Work out the finished part from the listing and answer in its coordinate system (mm). Face numbers are marked on the shaded views. Give positions to 0.01 mm unless a question says otherwise; leave off trailing zeros. Loops run counter-clockwise (first coordinate to the right, second up) from the corner with the lowest first, then second, coordinate; pieces in that order, holes last. Notation, with made-up numbers: (-1, -4.75) - (51, -4.75) arc R19 cw to (51, 28.25) - close; hole circle Ø5 at (23, 51.5). An arc over 180 degrees is marked (long way). One line per item, written item: value.
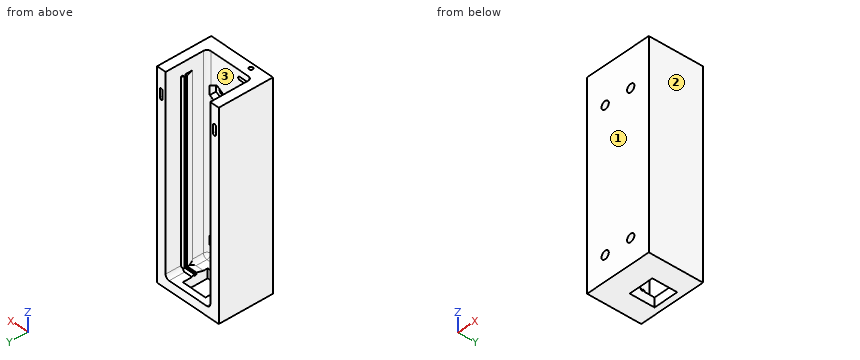
from build123d import *

# Parameters (mm, degrees)
BOSS_EXTRUDE1_DEPTH            = 82.55
BOSS_EXTRUDE2_START            = -5.08
BOSS_EXTRUDE2_DEPTH            = 77.47
BOSS_EXTRUDE4_REACH            = 89.467
SKETCH8_W                      = 27.6225
SKETCH8_H                      = 3.81
BOSS_EXTRUDE5_REACH            = 88.945
CUT_EXTRUDE1_REACH             = 86.753
SKETCH10_W                     = 10.16
SKETCH10_H                     = 10.16
SKETCH11_W                     = 27.6225
SKETCH11_H                     = 3.2766
CUT_EXTRUDE2_DEPTH             = 85.753025619
FILLET3_R                      = 1.5875
CUT_EXTRUDE3_DEPTH             = 2.286
CUT_EXTRUDE4_DEPTH             = 3.175
F_4_CLEARANCE_HOLE1_D          = 3.2639
CUT_EXTRUDE5_DEPTH             = 2.54
CUT_EXTRUDE5_DIRECTION_2_REACH = 87.415
SKETCH18_R                     = 0.762
CUT_EXTRUDE6_DEPTH             = 10.16


with BuildPart() as part:
    # Sketch1 → Boss-Extrude1 (new body)
    with BuildSketch(Plane.XY):
        Polygon((10.00125, 12.065), (10.00125, -8.255), (-10.00125, -8.255), (-10.00125, 12.065), (-13.81125, 12.065), (-13.81125, -13.335), (13.81125, -13.335), (13.81125, 12.065), align=None)
    extrude(amount=BOSS_EXTRUDE1_DEPTH)

    # Sketch3 → Boss-Extrude2 (add)
    with BuildSketch(Plane.XY.offset(82.55).offset(BOSS_EXTRUDE2_START)):
        Polygon((10.00125, 1.7018), (9.23925, 1.7018), (10.00125, 2.4638), align=None)
        Polygon((10.00125, 0.635), (9.23925, 0.635), (10.00125, -2.208822715), align=None)
        Polygon((-10.00125, 2.4638), (-10.00125, 1.7018), (-9.23925, 1.7018), align=None)
        Polygon((-10.00125, -2.208822715), (-10.00125, 0.635), (-9.23925, 0.635), align=None)
    extrude(amount=-BOSS_EXTRUDE2_DEPTH)

    # Boss-Extrude4: up to this face of the body (flat: up to its plane)
    boss_extrude4_end = Plane(part.part.faces().sort_by_distance((0, -8.255, 41.275))[0])
    # Sketch8 → Boss-Extrude4 (add, up to the picked face)
    with BuildSketch(Plane(origin=(0, 12.065, 0), x_dir=(1, 0, 0), z_dir=(0, 1, 0)), mode=Mode.PRIVATE) as boss_extrude4_sk1:
        with Locations((0, -1.905)):
            Rectangle(SKETCH8_W, SKETCH8_H)
    boss_extrude4_tool1 = split(extrude(boss_extrude4_sk1.sketch, amount=-BOSS_EXTRUDE4_REACH, mode=Mode.PRIVATE), bisect_by=boss_extrude4_end, keep=Keep.BOTH, mode=Mode.PRIVATE)
    add(boss_extrude4_tool1.solids().sort_by(Axis((0, 12.065, 1.905), (0, -1, 0)))[0])

    # Boss-Extrude5: up to this face of the body (flat: up to its plane)
    boss_extrude5_end = Plane(part.part.faces().sort_by_distance((10.00125, 7.2644, 4.623196778))[0])
    # Sketch9 → Boss-Extrude5 (add, up to the picked face)
    with BuildSketch(Plane(origin=(-10.00125, 0, 0), x_dir=(0, 0, -1), z_dir=(1, 0, 0)), mode=Mode.PRIVATE) as boss_extrude5_sk1:
        Polygon((-3.81, 2.4638), (-3.81, 1.7018), (-4.572, 1.7018), align=None)
    boss_extrude5_tool1 = split(extrude(boss_extrude5_sk1.sketch, amount=BOSS_EXTRUDE5_REACH, mode=Mode.PRIVATE), bisect_by=boss_extrude5_end, keep=Keep.BOTH, mode=Mode.PRIVATE)
    # Sketch9 → Boss-Extrude5 (add, up to the picked face)
    with BuildSketch(Plane(origin=(-10.00125, 0, 0), x_dir=(0, 0, -1), z_dir=(1, 0, 0)), mode=Mode.PRIVATE) as boss_extrude5_sk2:
        Polygon((-3.81, 0.635), (-3.81, -2.208822715), (-4.572, 0.635), align=None)
    boss_extrude5_tool2 = split(extrude(boss_extrude5_sk2.sketch, amount=BOSS_EXTRUDE5_REACH, mode=Mode.PRIVATE), bisect_by=boss_extrude5_end, keep=Keep.BOTH, mode=Mode.PRIVATE)
    add(boss_extrude5_tool1.solids().sort_by(Axis((-10.00125, 1.9558, 4.064), (1, 0, 0)))[0])
    add(boss_extrude5_tool2.solids().sort_by(Axis((-10.00125, -0.312941, 4.064), (1, 0, 0)))[0])

    # Sketch10 → Cut-Extrude1 (cut, up to next)
    with BuildSketch(Plane(origin=(0, 0, 0), x_dir=(-1, 0, 0), z_dir=(0, 0, -1)), mode=Mode.PRIVATE) as cut_extrude1_sk1:
        with Locations((0, 1.1684)):
            Rectangle(SKETCH10_W, SKETCH10_H)
    cut_extrude1_tool1 = extrude(cut_extrude1_sk1.sketch, amount=-CUT_EXTRUDE1_REACH, mode=Mode.PRIVATE) & part.part
    add(cut_extrude1_tool1.solids().sort_by_distance((0, 1.1684, 0))[0], mode=Mode.SUBTRACT)

    # Sketch11 → Cut-Extrude2 (cut, through all)
    with BuildSketch(Plane.XY.offset(82.55)):
        with Locations((0, 10.4267)):
            Rectangle(SKETCH11_W, SKETCH11_H)
    extrude(amount=-CUT_EXTRUDE2_DEPTH, mode=Mode.SUBTRACT)

    # Fillet3
    fillet3_edges = [part.edges().sort_by_distance(p)[0] for p in [
        (-10.00125, -8.255, 43.18),
        (10.00125, -8.255, 43.18),
        (10.00125, 5.6261, 3.81),
        (0, -8.255, 3.81),
        (10.00125, -5.231911358, 3.81),
        (-10.00125, 5.6261, 3.81),
        (-10.00125, -5.231911358, 3.81),
    ]]
    fillet(fillet3_edges, radius=FILLET3_R)

    # Sketch13 → Cut-Extrude3 (cut)
    with BuildSketch(Plane(origin=(0, -8.255, 0), x_dir=(1, 0, 0), z_dir=(0, 1, 0))):
        with BuildLine():
            Line((-7.651886934, -78.8162), (-4.476886934, -78.8162))
            ThreePointArc((-4.476886934, -78.8162), (-3.841886934, -79.4512), (-4.476886934, -80.0862))
            Line((-4.476886934, -80.0862), (-7.651886934, -80.0862))
            ThreePointArc((-7.651886934, -80.0862), (-8.286886934, -79.4512), (-7.651886934, -78.8162))
        make_face()
    extrude(amount=-CUT_EXTRUDE3_DEPTH, mode=Mode.SUBTRACT)

    # Sketch14 → Cut-Extrude4 (cut)
    with BuildSketch(Plane(origin=(0, 8.7884, 0), x_dir=(1, 0, 0), z_dir=(0, 1, 0))):
        with BuildLine():
            Line((-11.27125, -71.386954), (-11.27125, -74.561954))
            ThreePointArc((-11.27125, -74.561954), (-11.90625, -75.196954), (-12.54125, -74.561954))
            Line((-12.54125, -74.561954), (-12.54125, -71.386954))
            ThreePointArc((-12.54125, -71.386954), (-11.90625, -70.751954), (-11.27125, -71.386954))
        make_face()
        with BuildLine():
            Line((11.27125, -71.386954), (11.27125, -74.561954))
            ThreePointArc((11.27125, -74.561954), (11.90625, -75.196954), (12.54125, -74.561954))
            Line((12.54125, -74.561954), (12.54125, -71.386954))
            ThreePointArc((12.54125, -71.386954), (11.90625, -70.751954), (11.27125, -71.386954))
        make_face()
    extrude(amount=-CUT_EXTRUDE4_DEPTH, mode=Mode.SUBTRACT)

    # #4 Clearance Hole1 (through all)
    with Locations(Plane(origin=(0, -8.255, 0), x_dir=(1, 0, 0), z_dir=(0, 1, 0))):
        with Locations((-5.715, -10.16), (5.715, -67.31), (-5.715, -67.31), (5.715, -10.16)):
            Hole(F_4_CLEARANCE_HOLE1_D / 2)

    # Sketch17 → Cut-Extrude5 (cut)
    with BuildSketch(Plane(origin=(0, -8.255, 0), x_dir=(1, 0, 0), z_dir=(0, 1, 0))):
        Polygon((-5.715, -13.782180119), (-2.5781, -11.971090059), (-2.5781, -8.348909941), (-5.715, -6.537819881), (-8.8519, -8.348909941), (-8.8519, -11.971090059), align=None)
        Polygon((5.715, -13.782180119), (8.8519, -11.971090059), (8.8519, -8.348909941), (5.715, -6.537819881), (2.5781, -8.348909941), (2.5781, -11.971090059), align=None)
        Polygon((-5.715, -63.687819881), (-8.8519, -65.498909941), (-8.8519, -69.121090059), (-5.715, -70.932180119), (-2.5781, -69.121090059), (-2.5781, -65.498909941), align=None)
        Polygon((5.715, -63.687819881), (2.5781, -65.498909941), (2.5781, -69.121090059), (5.715, -70.932180119), (8.8519, -69.121090059), (8.8519, -65.498909941), align=None)
    extrude(amount=-CUT_EXTRUDE5_DEPTH, mode=Mode.SUBTRACT)

    # Sketch17 → Cut-Extrude5 direction 2 (cut, up to next)
    with BuildSketch(Plane(origin=(0, -8.255, 0), x_dir=(1, 0, 0), z_dir=(0, 1, 0)), mode=Mode.PRIVATE) as cut_extrude5_direction_2_sk1:
        Polygon((-5.715, -13.782180119), (-2.5781, -11.971090059), (-2.5781, -8.348909941), (-5.715, -6.537819881), (-8.8519, -8.348909941), (-8.8519, -11.971090059), align=None)
    cut_extrude5_direction_2_tool1 = extrude(cut_extrude5_direction_2_sk1.sketch, amount=CUT_EXTRUDE5_DIRECTION_2_REACH, mode=Mode.PRIVATE) & part.part
    # Sketch17 → Cut-Extrude5 direction 2 (cut, up to next)
    with BuildSketch(Plane(origin=(0, -8.255, 0), x_dir=(1, 0, 0), z_dir=(0, 1, 0)), mode=Mode.PRIVATE) as cut_extrude5_direction_2_sk2:
        Polygon((5.715, -13.782180119), (8.8519, -11.971090059), (8.8519, -8.348909941), (5.715, -6.537819881), (2.5781, -8.348909941), (2.5781, -11.971090059), align=None)
    cut_extrude5_direction_2_tool2 = extrude(cut_extrude5_direction_2_sk2.sketch, amount=CUT_EXTRUDE5_DIRECTION_2_REACH, mode=Mode.PRIVATE) & part.part
    # Sketch17 → Cut-Extrude5 direction 2 (cut, up to next)
    with BuildSketch(Plane(origin=(0, -8.255, 0), x_dir=(1, 0, 0), z_dir=(0, 1, 0)), mode=Mode.PRIVATE) as cut_extrude5_direction_2_sk3:
        Polygon((-5.715, -63.687819881), (-8.8519, -65.498909941), (-8.8519, -69.121090059), (-5.715, -70.932180119), (-2.5781, -69.121090059), (-2.5781, -65.498909941), align=None)
    cut_extrude5_direction_2_tool3 = extrude(cut_extrude5_direction_2_sk3.sketch, amount=CUT_EXTRUDE5_DIRECTION_2_REACH, mode=Mode.PRIVATE) & part.part
    # Sketch17 → Cut-Extrude5 direction 2 (cut, up to next)
    with BuildSketch(Plane(origin=(0, -8.255, 0), x_dir=(1, 0, 0), z_dir=(0, 1, 0)), mode=Mode.PRIVATE) as cut_extrude5_direction_2_sk4:
        Polygon((5.715, -63.687819881), (2.5781, -65.498909941), (2.5781, -69.121090059), (5.715, -70.932180119), (8.8519, -69.121090059), (8.8519, -65.498909941), align=None)
    cut_extrude5_direction_2_tool4 = extrude(cut_extrude5_direction_2_sk4.sketch, amount=CUT_EXTRUDE5_DIRECTION_2_REACH, mode=Mode.PRIVATE) & part.part
    add(cut_extrude5_direction_2_tool1.solids().sort_by_distance((-5.715, -8.255, 10.16))[0], mode=Mode.SUBTRACT)
    add(cut_extrude5_direction_2_tool2.solids().sort_by_distance((5.715, -8.255, 10.16))[0], mode=Mode.SUBTRACT)
    add(cut_extrude5_direction_2_tool3.solids().sort_by_distance((-5.715, -8.255, 67.31))[0], mode=Mode.SUBTRACT)
    add(cut_extrude5_direction_2_tool4.solids().sort_by_distance((5.715, -8.255, 67.31))[0], mode=Mode.SUBTRACT)

    # Sketch18 → Cut-Extrude6 (cut)
    with BuildSketch(Plane.XY.offset(82.55)):
        with Locations((-6.064467422, -11.430018288)):
            Circle(SKETCH18_R)
    extrude(amount=-CUT_EXTRUDE6_DEPTH, mode=Mode.SUBTRACT)


solid = part.part
1. Section D-D (z = 48) is taken. Write down the section's boundary in (x, y) (1 decimal).
Output:
outline: (-13.8, -13.3) - (13.8, -13.3) - (13.8, 8.8) - (10, 8.8) - (10, 2.5) - (9.2, 1.7) - (10, 1.7) - (10, 0.6) - (9.2, 0.6) - (10, -2.2) - (10, -6.7) arc R1.6 cw to (8.4, -8.3) - (-8.4, -8.3) arc R1.6 cw to (-10, -6.7) - (-10, -2.2) - (-9.2, 0.6) - (-10, 0.6) - (-10, 1.7) - (-9.2, 1.7) - (-10, 2.5) - (-10, 8.8) - (-13.8, 8.8) - close
2. Section C-C (y = -9.25) is taken. Count the separate pieces of the cut face and the enclosed holes in it, and give its area (3 significant figures).
Output:
separate pieces: 1
enclosed holes: 5
area: 2,140 mm²
3. Flat-ended cylindrical pins translate along their axes: pin 1 Ø7 at (x, z) = (-4.5, 11) entering from +Y (3 decimals); pin 2 Ø5 at (x, y) = (-3.5, -2.5) entering from +Z; pin 3 Ø5 at (x, z) = (5.715, 67.31) entering from +Y (3 decimals). Find the tip coordinate at first contact, or state that the pin passes through.
Output:
pin 1: stops at y = -8.255
pin 2: stops at z = 4.25
pin 3: stops at y = -10.795
4. The mould has two halves that part along X. Classify the marked faces 1, 2 and 3: released by +X, released by -X, zero draft, split by the parting line, or undercut.
Output:
face 1: zero draft
face 2: released by +X
face 3: undercut
5. Find the intervals of material crossed by line 1 along X through (y, z) = (-11.45, 67.31); line 2 along X through (y, z) = (-3, 57); line 3 along Y through (x, z) = (0, 9) (3 decimals), in increasing order.
Output:
line 1: x = -13.81 to -7.35, -4.08 to 4.08, 7.35 to 13.81
line 2: x = -13.81 to -10, 10 to 13.81
line 3: y = -13.335 to -8.255
